Autodesk Inventor part; units mm, degrees
ref_plane "YZ Plane" through (0, 0, 0) normal (1, 0, 0) x (0, 1, 0)
ref_plane "XZ Plane" through (0, 0, 0) normal (0, 1, 0) x (-1, 0, 0)
ref_plane "XY Plane" through (0, 0, 0) normal (0, 0, 1) x (1, 0, 0)
sketch "Sketch1" plane through (0, 0, 0) normal (0, 0, 1) x (1, 0, 0)
  line L0 (0, 0) -> (25.4, 0)
  line L1 (25.4, 0) -> (25.4, 38.1)
  line L2 (25.4, 38.1) -> (0, 38.1)
  line L3 (0, 38.1) -> (0, 0)
  line L4 (12.7, 38.1) -> (12.7, 0) construction
  circle A0 centre (12.7, 28.575) radius 3.302
  circle A1 centre (12.7, 9.525) radius 3.302
  dimension "d0" = 25.4
  dimension "d2" = 38.1
  dimension "d3" = 6.604
  dimension "d4" = 19.05
  dimension "d5" = 9.525
  dimension "d9" = 9.525
extrude "Extrusion1" add sketch "Sketch1" along normal blind 3.175
fillet "Fillet1" radius 3.175 4 edges at (25.4, 38.1, 1.5875) (0, 38.1, 1.5875) (25.4, 0, 1.5875) (0, 0, 1.5875)
properties part number "Chassis Tower Support Plate (for Bracket 1)" material "Aluminum 6061"
Part model, mm, in its own coordinate system. Round coordinates to 2 decimals unless told otherwise and drop trailing zeros. Write each loop counter-clockwise with the first axis right and the second up, starting at its lowest first coordinate (ties: lowest second). Pieces come first, ordered by that corner, then holes.
Item 1: Cut at D-D, the plane y = 27. Give the cut face in (x, z) (3 decimals), plus the area to 3 significant figures.
Results:
outline: (0, 0) - (9.798, 0) - (9.798, 3.175) - (0, 3.175) - close; (15.602, 0) - (25.4, 0) - (25.4, 3.175) - (15.602, 3.175) - close
area: 62.2 mm2
Item 2: Cut at A-A, the plane y = 9. Give the cut face in (x, z) (3 decimals), plus the area to 3 significant figures.
Results:
outline: (0, 0) - (9.44, 0) - (9.44, 3.175) - (0, 3.175) - close; (15.96, 0) - (25.4, 0) - (25.4, 3.175) - (15.96, 3.175) - close
area: 59.9 mm2
Item 3: Two-plate mould, pull along X, no slides. Class faces 1 (the flat face through (13, 19, 3.175)), 2 (the cylindrical face through (14.475, 6.741, 1.565)), 3 (the cylindrical face through (0.95, 37.19, 1.61)): +X half, -X half, draft (parallel to the pull), parting line (faces both ways), or undercut.
Results:
face 1: draft
face 2: undercut
face 3: -X half
Item 4: Cut at B-B, the plane x = 12.7. Give the cut face in (y, z) (3 decimals), plus the area to 3 significant figures.
Results:
outline: (0, 0) - (6.223, 0) - (6.223, 3.175) - (0, 3.175) - close; (12.827, 0) - (25.273, 0) - (25.273, 3.175) - (12.827, 3.175) - close; (31.877, 0) - (38.1, 0) - (38.1, 3.175) - (31.877, 3.175) - close
area: 79.0 mm2
Item 5: Drop a flat-ended pin along its axis: pin 1 Ø5.5 at (x, y) = (12.7, 9.525) entering from +Z. Give the stop position or say it passes through.
Results:
pin 1: passes through
Item 6: Probe L1, parallel to Y at x = 12.7, z = 2.3; L2, parallel to Y at x = 15.5, z = 2.25; L3, parallel to X at y = 10, z = 3. List the from-to ranges inside material, lowest first.
Results:
L1: y = 0 to 6.22, 12.83 to 25.27, 31.88 to 38.1
L2: y = 0 to 7.77, 11.28 to 26.82, 30.33 to 38.1
L3: x = 0 to 9.43, 15.97 to 25.4
Item 7: Cut at C-C, the plane z = 0.65. Give the cut face in (x, y) (3 decimals).
Results:
outline: (0, 3.175) arc R3.175 ccw to (3.175, 0) - (22.225, 0) arc R3.175 ccw to (25.4, 3.175) - (25.4, 34.925) arc R3.175 ccw to (22.225, 38.1) - (3.175, 38.1) arc R3.175 ccw to (0, 34.925) - close; hole circle Ø6.604 at (12.7, 9.525); hole circle Ø6.604 at (12.7, 28.575)
